```python
from build123d import *

# Parameters (mm, degrees)
SKETCH1_R           = 3.1
BOSS_EXTRUDE1_DEPTH = 5
SKETCH2_R           = 4.5
BOSS_EXTRUDE2_DEPTH = 2
SKETCH3_R           = 4.1
BOSS_EXTRUDE3_DEPTH = 8
CHAMFER1_SIZE       = 1


with BuildPart() as part:
    # Sketch1 → Boss-Extrude1 (new body)
    with BuildSketch(Plane(origin=(0, 0, 0), x_dir=(1, 0, 0), z_dir=(0, 1, 0))):
        with Locations(Location((0, 0, 0), (0, 0, 270))):
            Circle(SKETCH1_R)
    extrude(amount=BOSS_EXTRUDE1_DEPTH)

    # Sketch2 → Boss-Extrude2 (add)
    with BuildSketch(Plane(origin=(0, 3, 0), x_dir=(1, 0, 0), z_dir=(0, 1, 0))):
        with Locations(Location((0, 0, 0), (0, 0, 270))):
            Circle(SKETCH2_R)
    extrude(amount=BOSS_EXTRUDE2_DEPTH)

    # Sketch3 → Boss-Extrude3 (add)
    with BuildSketch(Plane(origin=(0, 5, 0), x_dir=(1, 0, 0), z_dir=(0, 1, 0))):
        with Locations(Location((0, 0, 0), (0, 0, 270))):
            Circle(SKETCH3_R)
    extrude(amount=BOSS_EXTRUDE3_DEPTH)

    # Chamfer1
    chamfer1_edges = [part.edges().sort_by_distance(p)[0] for p in [
        (0, 13, -4.1),
    ]]
    chamfer(chamfer1_edges, length=CHAMFER1_SIZE)


solid = part.part
```
Model file for the job. Use its own axes, mm. A direction names the side the tool comes from. Give positions to 0.01 mm unless a question says otherwise; leave off trailing zeros. Loops run counter-clockwise (first coordinate to the right, second up) from the corner with the lowest first, then second, coordinate; pieces in that order, holes last. Notation, with made-up numbers: (75.25, 3.25) - (123.25, 3.25) arc R7 ccw to (123.25, 15.25) - close; hole circle Ø5 at (12, 23.25). An arc over 180 degrees is marked (long way). One line per item, written item: value. Start each with the question number.
1. Slice it at A-A (x = 0). List the corners of the cut face in (y, z).
2. Which spindle directions (+Z, -Z, +X, -X, +Y, -Y) get a long thin tool onto all of the face, cutting with end or side? Do faces 1 (the flat face through (1.1, 3, -3.1)), 2 (the cylindrical face through (4.065, 8.451, -0.534)), 3 (the cylindrical face through (1.352, 3.986, 4.292)). Say none if no direction does.
3. Slice it at B-B (z = 0). List the corners of the cut face in (x, y), plus the area to 3 significant figures.
4. Pin check, flat tip, straight feed: pin 1 (3 mm diameter, centred on x = -2.5, y = 4, fed in from +Z). Stop position of the tip, or through.
5. Probe L1, parallel to Y at x = -3.5, z = -2.75; L2, parallel to Z at x = -2.75, y = 0.5; L3, parallel to X at y = 3.5, z = -1.25. List the from-to ranges inside material, lowest first. Write a range as from..to.
6. Slice it at C-C (y = 10). List the corners of the cut face in (x, z), plus the area to 3 significant figures.
Solution:
1. outline: (0, -3.1) - (3, -3.1) - (3, -4.5) - (5, -4.5) - (5, -4.1) - (12, -4.1) - (13, -3.1) - (13, 3.1) - (12, 4.1) - (5, 4.1) - (5, 4.5) - (3, 4.5) - (3, 3.1) - (0, 3.1) - close
2. face 1: -Y
2. face 2: +Y
2. face 3: +Y, -Y
3. outline: (-4.5, 3) - (-3.1, 3) - (-3.1, 0) - (3.1, 0) - (3.1, 3) - (4.5, 3) - (4.5, 5) - (4.1, 5) - (4.1, 12) - (3.1, 13) - (-3.1, 13) - (-4.1, 12) - (-4.1, 5) - (-4.5, 5) - close
3. area: 101 mm^2
4. pin 1: stops at z = 4.39
5. L1: y = 3..5
5. L2: z = -1.43..1.43
5. L3: x = -4.32..4.32
6. outline: circle Ø8.2 at (0, 0)
6. area: 52.8 mm^2
